Can you work these out from the model? Positions are in its coordinate system, mm. A direction names the side the tool comes from. Give positions to 0.01 mm unless a question says otherwise; leave off trailing zeros. Loops run counter-clockwise (first coordinate to the right, second up) from the corner with the lowest first, then second, coordinate; pieces in that order, holes last. Notation, with made-up numbers: (74.5, 6) - (103.5, 6) arc R20 ccw to (103.5, 14) - close; hole circle Ø11 at (72.25, -38). An arc over 180 degrees is marked (long way). Use a Markdown table: item, result. Add a question column.
```python
from build123d import *

# Parameters (mm, degrees)
EXTRUDE_1_DEPTH     = 5
SKETCH_2_R          = 1.5
EXTRUDE_2_DEPTH     = 8
SKETCH_3_R          = 1.5
CUT_EXTRUDE_1_DEPTH = 4
CHAMFER_1_SIZE      = 0.2
FILLET_1_R          = 0.1


with BuildPart() as part:
    # 草图1 → 凸台-拉伸1 (new body)
    with BuildSketch(Plane(origin=(0, 0, 0), x_dir=(1, 0, 0), z_dir=(0, 1, 0))):
        Polygon((2.713546265, 0), (1.356773133, 2.35), (-1.356773133, 2.35), (-2.713546265, 0), (-1.356773133, -2.35), (1.356773133, -2.35), align=None)
    extrude(amount=EXTRUDE_1_DEPTH)

    # 草图2 → 凸台-拉伸2 (add)
    with BuildSketch(Plane(origin=(0, 5, 0), x_dir=(1, 0, 0), z_dir=(0, 1, 0))):
        with Locations(Location((0, 0, 0), (0, 0, 270))):
            Circle(SKETCH_2_R)
    extrude(amount=EXTRUDE_2_DEPTH)

    # 草图3 → 切除-拉伸1 (cut)
    with BuildSketch(Plane.XZ):
        with Locations(Location((0, 0, 0), (0, 0, 90))):
            Circle(SKETCH_3_R)
    extrude(amount=-CUT_EXTRUDE_1_DEPTH, mode=Mode.SUBTRACT)

    # 倒角1
    chamfer_1_edges = [part.edges().sort_by_distance(p)[0] for p in [
        (0, 13, -1.5),
        (0, 4, -1.5),
    ]]
    chamfer(chamfer_1_edges, length=CHAMFER_1_SIZE)

    # 圆角1
    fillet_1_edges = [part.edges().sort_by_distance(p)[0] for p in [
        (1.356773133, 2.5, 2.35),
        (-1.356773133, 2.5, 2.35),
        (-2.713546265, 2.5, 0),
        (-1.356773133, 2.5, -2.35),
        (1.356773133, 2.5, -2.35),
        (2.713546265, 2.5, 0),
    ]]
    fillet(fillet_1_edges, radius=FILLET_1_R)


solid = part.part
```
1. On a 3-axis mill with a long thin cutter (end or side, diameter ignored), from which of +Z, -Z, +X, -X, +Y, -Y can I reach the whole of each face in a straight line? I mean faces 1 (the face through (-2.044, 2.465, 1.159)), 2 (the face through (0.45, 8.85, 1.43)). Say none if no direction works.
2. If we mould it in two halves opening along Z, with no side actions, what happens to faces 3 (the face through (2.026, 2.465, 1.191)), 4 (the face through (0, 4, 0)), 5 (the face through (0, 5, -2)), 6 (the face through (-0.45, 1.87, 1.43))? For each: released by +Z, released by -Z, zero draft, split by the parting line, or undercut.
3. Suppose I cut it at B-B (y = 7.25). List the corners of the cut face in (x, z) for me.
4. Will these pins go through, and if not, where does the flat tip stop? P1, Ø1, axis at y = 10.5, z = 0.5, coming from the -X side; P2, Ø2, axis at x = -1.5, y = 11.5, coming from the +Z side; P3, Ø0.8, axis at x = -0.5, z = 0.5, coming from the -Y side.
5. Suppose I cut it at D-D (x = -2). List the corners of the cut face in (y, z) for me.
6. Suppose I cut it at C-C (z = -2). List the corners of the cut face in (x, y) for me, and give its area (3 significant figures).
7. Suppose I cut it at A-A (x = 0). List the corners of the cut face in (y, z) for me.
8. Please list where these lines run through material, in increasing order: line 1 along X through (y, z) = (1.55, 0); line 2 along Y through (x, z) = (0.2, 1.6); line 3 along Y through (x, z) = (-0.85, 0.9). Write a range as [from, to].
Results below:
| question | item | result |
|---|---|---|
| 1 | face 1 | +Z, -X, +Y, -Y |
| 1 | face 2 | +Y |
| 2 | face 3 | released by +Z |
| 2 | face 4 | undercut |
| 2 | face 5 | zero draft |
| 2 | face 6 | undercut |
| 3 | outline | circle Ø3 at (0, 0) |
| 4 | P1 | x = -1.5 |
| 4 | P2 | z = 1.41 |
| 4 | P3 | y = 4 |
| 5 | outline | (0, -1.24) - (5, -1.24) - (5, 1.24) - (0, 1.24) - close |
| 6 | outline | (-1.56, 0) - (1.56, 0) - (1.56, 5) - (-1.56, 5) - close |
| 6 | area | 15.6 mm² |
| 7 | outline | (0, -2.35) - (5, -2.35) - (5, -1.5) - (12.8, -1.5) - (13, -1.3) - (13, 1.3) - (12.8, 1.5) - (5, 1.5) - (5, 2.35) - (0, 2.35) - (0, 1.5) - (3.8, 1.5) - (4, 1.3) - (4, -1.3) - (3.8, -1.5) - (0, -1.5) - close |
| 8 | line 1 | [-2.7, -1.5], [1.5, 2.7] |
| 8 | line 2 | [0, 5] |
| 8 | line 3 | [4, 13] |
